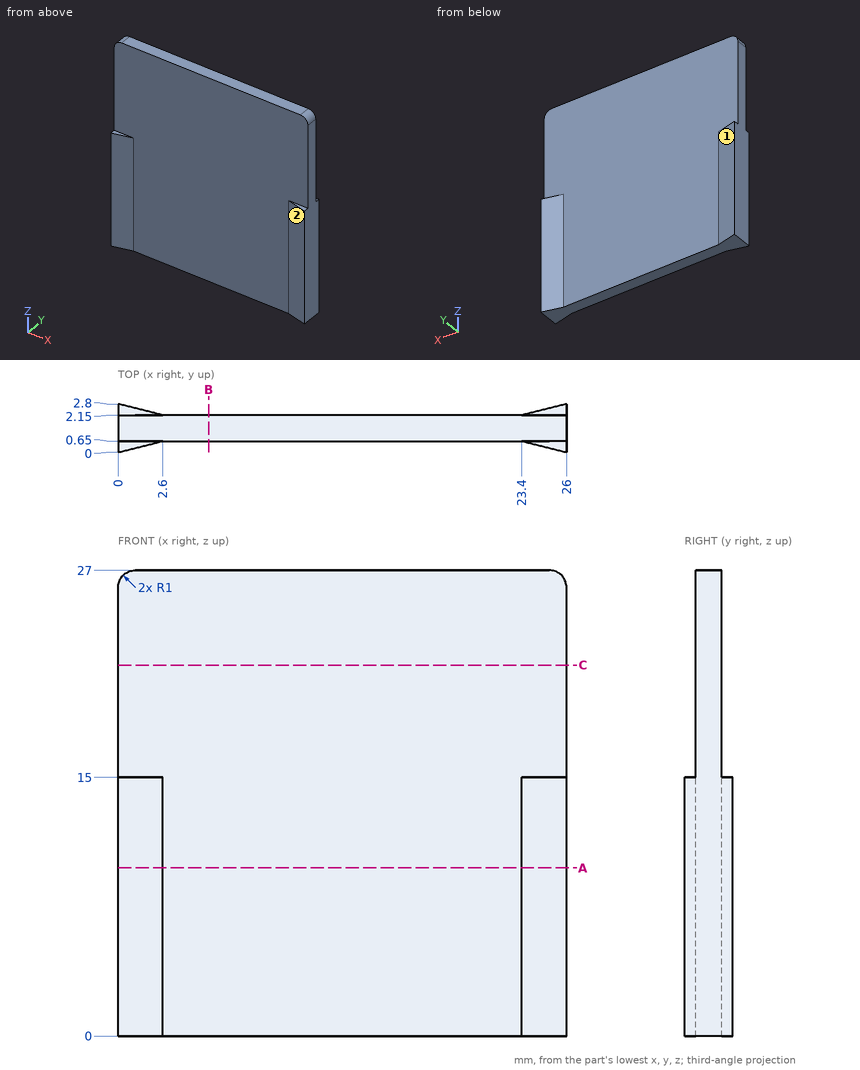
Check sheet for the drawn part. Datum: minimum x, y, z corner. Units: mm. A direction names the side the tool comes from. Give positions to 0.01 mm unless a question says otherwise; leave off trailing zeros. Loops run counter-clockwise (first coordinate to the right, second up) from the corner with the lowest first, then second, coordinate; pieces in that order, holes last. Notation, with made-up numbers: (27.25, 17.25) - (39.25, 17.25) arc R31 ccw to (39.25, 49.25) - close; hole circle Ø6 at (74, 89). An arc over 180 degrees is marked (long way). Write each question's results on one line, items separated by ' | '.
1) Tool access check on the marked faces 1 and 2. Record the directions out of +Z, -Z, +X, -X, +Y, -Y that give a thin tool (end or side, any length) a straight path to the whole face; none if there is none.
Solution:
face 1: +Z, -Z, +Y | face 2: +Z, -Z, -Y
2) Depth check by flat-ended pin: P1, Ø8, axis at x = 10.5, z = 7.5, coming from the +Y side. Enter the tip coordinate at first touch or a pass-through.
Solution:
P1: y = 2.15
3) Sectioned sample at C-C on z = 21.5. Record the boundary of the cut face in (x, y).
Solution:
outline: (0, 0.65) - (26, 0.65) - (26, 2.15) - (0, 2.15) - close
4) Sectioned sample at A-A on z = 9.75. Record the boundary of the cut face in (x, y).
Solution:
outline: (0, 0) - (2.6, 0.65) - (23.4, 0.65) - (26, 0) - (26, 2.8) - (23.4, 2.15) - (2.6, 2.15) - (0, 2.8) - close
5) Material ranges on L1, parallel to Y at x = 15.75, z = 13.5; L2, parallel to Y at x = 24.5, z = 10.5 (3 decimals), recorded low to high. Write a range as from..to.
Solution:
L1: 0.65..2.15 | L2: 0.375..2.425
6) Sectioned sample at B-B on x = 5.25. Record the boundary of the cut face in (y, z), plus the area to 3 significant figures.
Solution:
outline: (0.65, 0) - (2.15, 0) - (2.15, 27) - (0.65, 27) - close | area: 40.5 mm2
